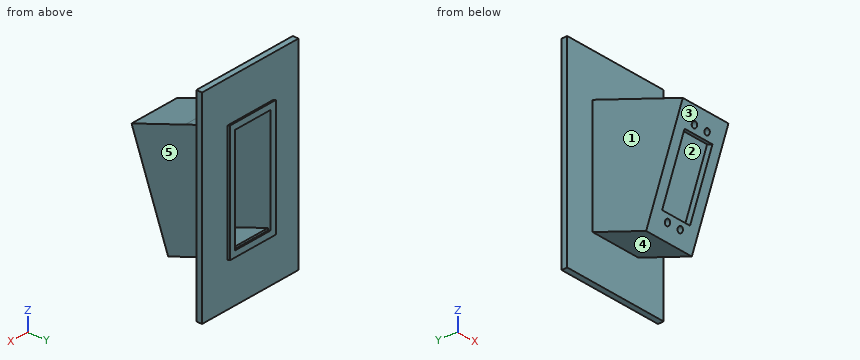
```python
from build123d import *

# Parameters (mm, degrees)
BOSS_EXTRU_1_DEPTH      = 18
BOSS_EXTRU_4_DEPTH      = 1
COQUE7_START            = 2
COQUE7_DEPTH            = 14
ESQUISSE2_R             = 1
ESQUISSE2_W             = 11
ESQUISSE2_H             = 23
ENL_V_MAT_EXTRU_1_DEPTH = 69.486359517
ESQUISSE7_W             = 70
ESQUISSE7_H             = 2
BOSS_EXTRU_5_DEPTH      = 10
ESQUISSE8_W             = 70
ESQUISSE8_H             = 2
BOSS_EXTRU_6_DEPTH      = 10


# Read off the part's stored shape, not the designer's step: Coque7
with BuildPart() as part:
    # Esquisse1 → Boss.-Extru.1 (new body)
    with BuildSketch(Plane(origin=(0, 0, 0), x_dir=(0, 0, -1), z_dir=(1, 0, 0))):
        Polygon((-35.320888862, -14.855752194), (-40, -2), (-55, -2), (-55, 0), (-40, 0), (0, 0), (15, 0), (15, -2), (0, -2), (6.840402867, -20.793852416), (-28.480485996, -33.649604609), align=None)
    extrude(amount=BOSS_EXTRU_1_DEPTH)

    # Esquisse3D1 → Boss.-Extru.4 (add, along a direction that is not the sketch's normal)
    with BuildSketch(Plane(origin=(0, 0, 0), x_dir=(0.40423775033266973, 0, 0.9146539461490243), z_dir=(0, -1, 0))):
        Polygon((0, 0), (37.251971468, 16.463771031), (44.528250974, 0), (7.276279506, -16.463771031), align=None)
    extrude(amount=-BOSS_EXTRU_4_DEPTH, dir=(0, -0.9396926207859081, -0.3420201433256695))

    # Coque7 outline → Coque7 (cut)
    with BuildSketch(Plane.YZ.offset(COQUE7_START)):
        Polygon((0, 2.856296013), (0, 2.128355545), (0.939692621, 2.470375688), (0.939692621, 38.941605067), (-31.086179081, 27.285141041), (-19.598507461, -4.276977338), align=None)
    extrude(amount=COQUE7_DEPTH, mode=Mode.SUBTRACT)

    # Esquisse2 → Enlèv. mat.-Extru.1 (cut, through all)
    with BuildSketch(Plane(origin=(0, -20.559896859, -7.483190476), x_dir=(1, 0, 0), z_dir=(0, -0.9396926207859082, -0.34202014332566943))):
        with Locations(Location((6.5, 33.277892702, 0), (0, 0, 270))):
            Circle(ESQUISSE2_R)
        with Locations(Location((11.5, 33.277892702, 0), (0, 0, 90))):
            Circle(ESQUISSE2_R)
        with Locations(Location((11.5, 5.677892702, 0), (0, 0, 270))):
            Circle(ESQUISSE2_R)
        with Locations(Location((6.5, 5.677892702, 0), (0, 0, 90))):
            Circle(ESQUISSE2_R)
        with Locations((9, 19.477892702)):
            Rectangle(ESQUISSE2_W, ESQUISSE2_H)
    extrude(amount=-ENL_V_MAT_EXTRU_1_DEPTH, mode=Mode.SUBTRACT)

    # Esquisse7 → Boss.-Extru.5 (add)
    with BuildSketch(Plane.ZY):
        with Locations((20, -1)):
            Rectangle(ESQUISSE7_W, ESQUISSE7_H)
    extrude(amount=BOSS_EXTRU_5_DEPTH)

    # Esquisse8 → Boss.-Extru.6 (add)
    with BuildSketch(Plane(origin=(18, 0, 0), x_dir=(0, 0, -1), z_dir=(1, 0, 0))):
        with Locations((-20, -1)):
            Rectangle(ESQUISSE8_W, ESQUISSE8_H)
    extrude(amount=BOSS_EXTRU_6_DEPTH)


solid = part.part
```
Input: part model. Units: mm. Frame: model coordinates. Face numbers are marked on the shaded views. A direction names the side the tool comes from. Give positions to 0.01 mm unless a question says otherwise; leave off trailing zeros. Loops run counter-clockwise (first coordinate to the right, second up) from the corner with the lowest first, then second, coordinate; pieces in that order, holes last.
1) Section query C-C on x = 17. Return the cut outline in (y, z), and give its area (3 significant figures).
A:
outline: (-33.65, 28.48) - (-20.79, -6.84) - (-2, 0) - (-2, -15) - (0, -15) - (0, 0) - (0.94, 0.34) - (0.94, 41.07) - (0, 40.73) - (0, 55) - (-2, 55) - (-2, 40) - close
area: 1,190 mm2
2) Section query B-B on x = 8.5. Return the cut outline in (y, z), and give its area (3 significant figures).
A:
outline: (-33.65, 28.48) - (-31.15, 21.63) - (-29.28, 22.31) - (-31.09, 27.29) - (0.94, 38.94) - (0.94, 41.07) - (0, 40.73) - (0, 55) - (-2, 55) - (-2, 40) - close; (-23.29, 0.01) - (-20.79, -6.84) - (-2, 0) - (-2, -15) - (0, -15) - (0, 0) - (0.94, 0.34) - (0.94, 2.47) - (0, 2.13) - (0, 2.86) - (-19.6, -4.28) - (-21.41, 0.7) - close
area: 201 mm2
3) Mould query, pull axis X, two halves, no side actions, for the marked faces 1, 2 and 3. Classes: released by +X, released by -X, zero draft, split by the parting line, or undercut.
A:
face 1: released by -X
face 2: undercut
face 3: zero draft
4) Section query A-A on z = 16. Return the cut outline in (x, y).
A:
outline: (-10, -2) - (0, -2) - (0, -29.11) - (3.5, -29.11) - (3.5, -26.98) - (2, -26.98) - (2, 0.94) - (0, 0.94) - (0, 0) - (-10, 0) - close; (14.5, -29.11) - (18, -29.11) - (18, -2) - (28, -2) - (28, 0) - (18, 0) - (18, 0.94) - (16, 0.94) - (16, -26.98) - (14.5, -26.98) - close
5) Contact query for flat-ended pins moving along their axis: pin 1 (16 mm diameter, centred on y = -15.5, z = 25.5, fed in from +X); pin 2 (4 mm diameter, centred on x = 3, y = -28.5, fed in from +Z); pin 3 (3 mm diameter, centred on y = -13.5, z = 2.5, fed in from -X); pin 4 (0.8 mm diameter, centred on x = 8.5, z = 2.5, fed in from +Y). Output: stop coordinate, or through.
A:
pin 1: stops at x = 18
pin 2: stops at z = 31.08
pin 3: stops at x = 0
pin 4: stops at y = 0.94
6) Section query D-D on y = -27. Return the cut outline in (x, z).
A:
outline: (0, 10.21) - (3.5, 10.21) - (3.5, 16.06) - (2, 16.06) - (2, 28.77) - (16, 28.77) - (16, 16.06) - (14.5, 16.06) - (14.5, 10.21) - (18, 10.21) - (18, 30.9) - (0, 30.9) - close
7) Line query: L1, parallel to X at y = -13.5, z = 28; L2, parallel to X at y = -1.5, z = 13.5; L3, parallel to Y at x = 18.5, z = 3.5. Output: solid intervals per line, ascending.
A:
L1: x = 0 to 2, 16 to 18
L2: x = -10 to 2, 16 to 28
L3: y = -2 to 0
8) Reachability of the marked faces 4 and 5 from +Z, -Z, +X, -X, +Y, -Y: full face, straight path, thin tool, end or side. Return the list, or none.
A:
face 4: -Z, +X, -X
face 5: +Z, -Z, +X, -Y
